from build123d import *

# Parameters (mm, degrees)
SKETCH1_W           = 50
SKETCH1_H           = 77.4
SKETCH1_R           = 2
BOSS_EXTRUDE1_DEPTH = 3
SKETCH2_R           = 1.75
BOSS_EXTRUDE2_DEPTH = 17
SKETCH3_W           = 50
SKETCH3_H           = 16
BOSS_EXTRUDE3_DEPTH = 3.5
SKETCH6_W           = 30
SKETCH6_H           = 16
CUT_EXTRUDE3_DEPTH  = 3.5


with BuildPart() as part:
    # Sketch1 → Boss-Extrude1 (new body)
    with BuildSketch(Plane(origin=(15, 0, 0), x_dir=(0, 0, -1), z_dir=(1, 0, 0))):
        with Locations((-55.110705908, 0)):
            Rectangle(SKETCH1_W, SKETCH1_H)
        with Locations((-55.110705908, 20.7)):
            Circle(SKETCH1_R, mode=Mode.SUBTRACT)
        with Locations(Location((-55.110705908, -20.7, 0), (0, 0, 180))):
            Circle(SKETCH1_R, mode=Mode.SUBTRACT)
    extrude(amount=-BOSS_EXTRUDE1_DEPTH)

    # Sketch2 → Boss-Extrude2 (add)
    with BuildSketch(Plane.ZY.offset(-12)):
        with BuildLine():
            Line((30.110705908, 38.7), (80.110705908, 38.7))
            Line((80.110705908, 38.7), (80.110705908, 28.7))
            Line((80.110705908, 28.7), (67.799283448, 28.7))
            ThreePointArc((67.799283448, 28.7), (55.110705908, 35.7), (42.422128367, 28.7))
            Line((42.422128367, 28.7), (30.110705908, 28.7))
            Line((30.110705908, 28.7), (30.110705908, 38.7))
        make_face()
        with Locations((34.110705908, 33.7)):
            Circle(SKETCH2_R, mode=Mode.SUBTRACT)
        with Locations((41.110705908, 33.7)):
            Circle(SKETCH2_R, mode=Mode.SUBTRACT)
        with Locations((69.110705908, 33.7)):
            Circle(SKETCH2_R, mode=Mode.SUBTRACT)
        with Locations((76.110705908, 33.7)):
            Circle(SKETCH2_R, mode=Mode.SUBTRACT)
    boss_extrude2 = extrude(amount=BOSS_EXTRUDE2_DEPTH)

    # Mirror1: Boss-Extrude2 across plane
    add(boss_extrude2.mirror(Plane.ZX))

    # Sketch3 → Boss-Extrude3 (add)
    with BuildSketch(Plane.ZY.offset(-12)):
        with Locations((55.110705908, 0)):
            Rectangle(SKETCH3_W, SKETCH3_H)
    extrude(amount=BOSS_EXTRUDE3_DEPTH)

    # Sketch6 → Cut-Extrude3 (cut)
    with BuildSketch(Plane.ZY.offset(-8.5)):
        with Locations((55.110705908, 0)):
            Rectangle(SKETCH6_W, SKETCH6_H)
    extrude(amount=-CUT_EXTRUDE3_DEPTH, mode=Mode.SUBTRACT)

    # loft from a face of the part (loft2)
    loft([part.faces().sort_by_distance((3.5, 28.7, 36.266417138))[0], part.faces().sort_by_distance((10.25, 8, 35.110705908))[0]])

    # loft from a face of the part (loft3)
    loft([part.faces().sort_by_distance((10.25, 8, 75.110705908))[0], part.faces().sort_by_distance((3.5, 28.7, 73.954994678))[0]])

    # loft from a face of the part (loft4)
    loft([part.faces().sort_by_distance((10.25, -8, 35.110705908))[0], part.faces().sort_by_distance((3.5, -28.7, 36.266417138))[0]])

    # loft from a face of the part (loft5)
    loft([part.faces().sort_by_distance((3.5, -28.7, 73.954994678))[0], part.faces().sort_by_distance((10.25, -8, 75.110705908))[0]])


solid = part.part
Can you work these out from the model? Positions are in its coordinate system, mm. A direction names the side the tool comes from. Give positions to 0.01 mm unless a question says otherwise; leave off trailing zeros. Order: outer loops, then holes, each group sorted by start corner. A loop starts at its lowest first (then second) coordinate and runs counter-clockwise, first axis right, second up. Notation, with made-up numbers: M 76,16 L 126,16 A32 cw 126,50 Z; hole C 71,62.25 d6. An arc over 180 degrees is marked long. Use one line per item in the form item = value. Start each with the question number.
Item 1: Will these pins go through, and if not, where does the flat tip stop? pin 1 Ø12 at (x, y) = (-1, -11) entering from +Z; pin 2 Ø1 at (y, z) = (34, 75.5) entering from -X; pin 3 Ø11 at (y, z) = (3, 33.5) entering from -X.
Item 2: If we section it at A-A (y = -1): Write out the boundary of the cut face in (x, z).
Item 3: If we section it at D-D (y = -33.7): Write out the boundary of the cut face in (x, z).
Item 4: For faces 4 (the flat face through (12, 34, 69)), 5 (the flat face through (-5, -36, 55)), which set-ups out of +Z, -Z, +X, -X, +Y, -Y let a thin tool reach every point of the face, with its end or its side?
Item 5: If I drill on line 1 along Y through (x, z) = (8, 75); line 2 along Z through (x, y) = (14.25, -20.7); line 3 along Y through (x, z) = (2.5, 69.5), over which ranges is the centre line in solid material (lowest first)?
Item 6: If we section it at B-B (x = 7): State how many separate pieces and enclosed holes the cut face has, then the cut area to 3 significant figures.
Item 7: If we section it at C-C (z = 51.5): Write out the boundary of the cut face in (x, y).
Item 8: We'd pull the mould along Z, two halves only. Please class faces 1 (the flat face through (10, 1, 30.111)), 2 (the flat face through (10, 0, 40.111)), 3 (the flat face through (15, 1, 55)): +Z half, -Z half, draft (parallel to the pull), parting line (faces both ways), or undercut.
Outcome:
q1.pin_1 = through
q1.pin_2 = 12
q1.pin_3 = 8.17
q2.outline = M 8.5,30.11 L 15,30.11 L 15,80.11 L 8.5,80.11 L 8.5,70.11 L 12,70.11 L 12,40.11 L 8.5,40.11 Z
q3.outline = M -5,30.11 L 15,30.11 L 15,80.11 L -5,80.11 L -5,77.86 L 12,77.86 L 12,74.36 L -5,74.36 L -5,70.86 L 12,70.86 L 12,67.36 L -5,67.36 L -5,62.59 L 12,62.59 L 12,47.63 L -5,47.63 L -5,42.86 L 12,42.86 L 12,39.36 L -5,39.36 L -5,35.86 L 12,35.86 L 12,32.36 L -5,32.36 Z
q4.face_4 = -X
q4.face_5 = +Z, -Z, -X, +Y, -Y
q5.line_1 = -38.7 to -35.05, -32.35 to -8.77, 8.77 to 32.35, 35.05 to 38.7
q5.line_2 = 30.11 to 53.11, 57.11 to 80.11
q5.line_3 = -38.7 to -35.41, -31.99 to -17.2, 17.2 to 31.99, 35.41 to 38.7
q6.separate_pieces = 2
q6.enclosed_holes = 8
q6.area = 1,500 mm2
q7.outline = M -5,-38.7 L 15,-38.7 L 15,38.7 L -5,38.7 L -5,35.26 L 12,35.26 L 12,-35.26 L -5,-35.26 Z
q8.face_1 = -Z half
q8.face_2 = undercut
q8.face_3 = draft
